```python
from build123d import *

# Parameters (mm, degrees)
PAD_DEPTH       = 19
POCKET_DEPTH    = 8.001
PAD001_DEPTH    = 12
SKETCH003_W     = 3.5
SKETCH003_H     = 0.4
POCKET001_DEPTH = 0.4
SKETCH004_W     = 5
SKETCH004_H     = 0.4
POCKET002_DEPTH = 0.4
SKETCH005_W     = 1.9
SKETCH005_H     = 0.4
POCKET003_DEPTH = 0.4
SKETCH006_W     = 5.1
SKETCH006_H     = 0.4
POCKET004_DEPTH = 0.4
SKETCH007_W     = 1.7
SKETCH007_H     = 0.4
POCKET005_DEPTH = 0.4
SKETCH008_W     = 7.2
SKETCH008_H     = 0.4
POCKET006_DEPTH = 0.4
SKETCH009_W     = 3
SKETCH009_H     = 0.8
PAD002_DEPTH    = 7
SKETCH010_W     = 3
SKETCH010_H     = 0.4
POCKET007_DEPTH = 0.4


with BuildPart() as part:
    # Sketch → Pad (new body)
    with BuildSketch(Plane.XY):
        Polygon((-25.168114, 28.93024), (-17.168114, 28.93024), (-17.168114, 23.93024), (-19.668114, 23.93024), (-19.668114, 25.43024), (-22.168114, 25.43024), (-22.168114, -0.06976), (-25.168114, -0.06976), align=None)
    extrude(amount=PAD_DEPTH)

    # Sketch001 → Pocket (cut, through all)
    with BuildSketch(Plane(origin=(-25.168114, 0, 0), x_dir=(0, -1, 0), z_dir=(-1, 0, 0))):
        Polygon((-28.93024, 15.5), (-9.93024, 15.5), (-9.93024, 12.75), (-2.93024, 12.75), (-2.93024, 6.25), (-9.93024, 6.25), (-9.93024, 3.5), (-28.93024, 3.5), align=None)
    extrude(amount=-POCKET_DEPTH, mode=Mode.SUBTRACT)

    # Sketch002 → Pad001 (new body)
    with BuildSketch(Plane.XY.offset(3.5)):
        Polygon((-25.168114, 28.93024), (-17.168114, 28.93024), (-17.168114, 23.93024), (-19.668114, 23.93024), (-19.668114, 25.43024), (-25.168114, 25.43024), align=None)
        Polygon((-24.368114, 26.23024), (-24.368114, 28.13024), (-17.968114, 28.13024), (-17.968114, 24.73024), (-18.868114, 24.73024), (-18.868114, 26.23024), align=None, mode=Mode.SUBTRACT)
    extrude(amount=PAD001_DEPTH)

    # Sketch003 → Pocket001 (cut)
    with BuildSketch(Plane(origin=(-25.168114, 0, 0), x_dir=(0, -1, 0), z_dir=(-1, 0, 0))):
        with Locations((-27.18024, 15.3)):
            Rectangle(SKETCH003_W, SKETCH003_H)
        with Locations((-27.18024, 3.7)):
            Rectangle(SKETCH003_W, SKETCH003_H)
    extrude(amount=-POCKET001_DEPTH, mode=Mode.SUBTRACT)

    # Sketch004 → Pocket002 (cut)
    with BuildSketch(Plane.YZ.offset(-17.168114)):
        with Locations((26.43024, 15.3)):
            Rectangle(SKETCH004_W, SKETCH004_H)
        with Locations((26.43024, 3.7)):
            Rectangle(SKETCH004_W, SKETCH004_H)
    extrude(amount=-POCKET002_DEPTH, mode=Mode.SUBTRACT)

    # Sketch005 → Pocket003 (cut)
    with BuildSketch(Plane(origin=(-19.668114, 0, 0), x_dir=(0, -1, 0), z_dir=(-1, 0, 0))):
        with Locations((-24.88024, 15.3)):
            Rectangle(SKETCH005_W, SKETCH005_H)
        with Locations((-24.88024, 3.7)):
            Rectangle(SKETCH005_W, SKETCH005_H)
    extrude(amount=-POCKET003_DEPTH, mode=Mode.SUBTRACT)

    # Sketch006 → Pocket004 (cut)
    with BuildSketch(Plane.XZ.offset(-25.43024)):
        with Locations((-22.218114, 15.3)):
            Rectangle(SKETCH006_W, SKETCH006_H)
        with Locations((-22.218114, 3.7)):
            Rectangle(SKETCH006_W, SKETCH006_H)
    extrude(amount=-POCKET004_DEPTH, mode=Mode.SUBTRACT)

    # Sketch007 → Pocket005 (cut)
    with BuildSketch(Plane.XZ.offset(-23.93024)):
        with Locations((-18.418114, 15.3)):
            Rectangle(SKETCH007_W, SKETCH007_H)
        with Locations((-18.418114, 3.7)):
            Rectangle(SKETCH007_W, SKETCH007_H)
    extrude(amount=-POCKET005_DEPTH, mode=Mode.SUBTRACT)

    # Sketch008 → Pocket006 (cut)
    with BuildSketch(Plane(origin=(0, 28.93024, 0), x_dir=(-1, 0, 0), z_dir=(0, 1, 0))):
        with Locations((21.168114, 15.3)):
            Rectangle(SKETCH008_W, SKETCH008_H)
        with Locations((21.168114, 3.7)):
            Rectangle(SKETCH008_W, SKETCH008_H)
    extrude(amount=-POCKET006_DEPTH, mode=Mode.SUBTRACT)

    # Sketch009 → Pad002 (new body)
    with BuildSketch(Plane.XY.offset(6.25)):
        with Locations((-23.668114, 9.53024)):
            Rectangle(SKETCH009_W, SKETCH009_H)
    extrude(amount=PAD002_DEPTH)

    # Sketch010 → Pocket007 (cut)
    with BuildSketch(Plane.XZ.offset(-9.13024)):
        with Locations((-23.668114, 12.55)):
            Rectangle(SKETCH010_W, SKETCH010_H)
        with Locations((-23.668114, 6.45)):
            Rectangle(SKETCH010_W, SKETCH010_H)
    extrude(amount=-POCKET007_DEPTH, mode=Mode.SUBTRACT)


solid = part.part
```
Input: part model. Units: mm. Frame: model coordinates. A direction names the side the tool comes from. Round coordinates to 2 decimals unless told otherwise and drop trailing zeros. Write each loop counter-clockwise with the first axis right and the second up, starting at its lowest first coordinate (ties: lowest second). Pieces come first, ordered by that corner, then holes. Notation, with made-up numbers: (46.5, 62.5) -> (91.5, 62.5) arc R15 ccw to (91.5, 70.5) -> close; hole circle Ø10 at (80, 1.5). An arc over 180 degrees is marked (long way). Answer as CSV lines item,"result".
1. Reachability of faces 1 (the flat face through (-19.668, 25, 2)), 2 (the flat face through (-19.668, 25, 9)), 3 (the flat face through (-18.4, 24.73, 9.4)), 4 (the flat face through (-22, 25.43, 9)) from +Z, -Z, +X, -X, +Y, -Y: full face, straight path, thin tool, end or side. Return the list, or none.
Geometry says:
face 1,"+Z, -Z, -Y"
face 2,"+Z, -Z, -X, -Y"
face 3,"none"
face 4,"-X"
2. Section C-C (z = 8). Return the cut outline in (x, y), plus the area to 3 significant figures.
Geometry says:
outline,"(-25.17, -0.07) -> (-22.17, -0.07) -> (-22.17, 2.93) -> (-25.17, 2.93) -> close; (-25.17, 9.13) -> (-22.17, 9.13) -> (-22.17, 9.93) -> (-25.17, 9.93) -> close; (-25.17, 25.43) -> (-19.67, 25.43) -> (-19.67, 23.93) -> (-17.17, 23.93) -> (-17.17, 28.93) -> (-25.17, 28.93) -> close; hole (-24.37, 26.23) -> (-18.87, 26.23) -> (-18.87, 24.73) -> (-17.97, 24.73) -> (-17.97, 28.13) -> (-24.37, 28.13) -> close"
area,"29.6 mm^2"
3. Section B-B (y = 12.25). Return the cut outline in (x, z).
Geometry says:
outline,"(-25.17, 0) -> (-22.17, 0) -> (-22.17, 3.5) -> (-25.17, 3.5) -> close; (-25.17, 15.5) -> (-22.17, 15.5) -> (-22.17, 19) -> (-25.17, 19) -> close"
4. Section A-A (z = 14.5). Return the cut outline in (x, y), plus the area to 3 significant figures.
Geometry says:
outline,"(-25.17, -0.07) -> (-22.17, -0.07) -> (-22.17, 9.93) -> (-25.17, 9.93) -> close; (-25.17, 25.43) -> (-19.67, 25.43) -> (-19.67, 23.93) -> (-17.17, 23.93) -> (-17.17, 28.93) -> (-25.17, 28.93) -> close; hole (-24.37, 26.23) -> (-18.87, 26.23) -> (-18.87, 24.73) -> (-17.97, 24.73) -> (-17.97, 28.13) -> (-24.37, 28.13) -> close"
area,"48.2 mm^2"
5. Ray query, L1, parallel to Z at x = -22.75, y = 25.75; L2, parallel to Y at x = -22.75, z = 12; L3, parallel to Z at x = -24.5, y = 3. Return the intervals inside material, ascending. Write a range as [from, to].
Geometry says:
L1,"z = [0, 3.5], [3.9, 15.1], [15.5, 19]"
L2,"y = [-0.07, 2.93], [9.13, 9.93], [25.43, 26.23], [28.13, 28.93]"
L3,"z = [0, 6.25], [12.75, 19]"
6. Mould query, pull axis Z, two halves, no side actions, for faces 5 (the flat face through (-22.168, 9.7, 9.4)), 6 (the flat face through (-23, 18, 0)), 7 (the flat face through (-24, 9.93, 9)). Classes: +Z half, -Z half, draft (parallel to the pull), parting line (faces both ways), or undercut.
Geometry says:
face 5,"draft"
face 6,"-Z half"
face 7,"undercut"
7. Section D-D (x = -21). Return the cut outline in (y, z), plus the area to 3 significant figures.
Geometry says:
outline,"(25.43, 0) -> (28.93, 0) -> (28.93, 3.5) -> (28.53, 3.5) -> (28.53, 3.9) -> (28.93, 3.9) -> (28.93, 15.1) -> (28.53, 15.1) -> (28.53, 15.5) -> (28.93, 15.5) -> (28.93, 19) -> (25.43, 19) -> (25.43, 15.5) -> (25.83, 15.5) -> (25.83, 15.1) -> (25.43, 15.1) -> (25.43, 3.9) -> (25.83, 3.9) -> (25.83, 3.5) -> (25.43, 3.5) -> close; hole (26.23, 3.5) -> (28.13, 3.5) -> (28.13, 15.5) -> (26.23, 15.5) -> close"
area,"43.1 mm^2"
8. Contact query for a flat-ended pin moving along its axis: P1, Ø2, axis at x = -19, z = 8, coming from the -Y side. Output: stop coordinate, or through.
Geometry says:
P1,"stops at y = 23.93"
